Verification items for this drawing (mm, ordinates from the low corner). Round coordinates to 2 decimals unless told otherwise and drop trailing zeros. Loops run counter-clockwise (first coordinate to the right, second up) from the corner with the lowest first, then second, coordinate; pieces in that order, holes last. Notation, with made-up numbers: (13, -10) -> (42, -10) arc R23 ccw to (42, 2) -> close; hole circle Ø10 at (-32.5, 30.25). An arc over 180 degrees is marked (long way). Use a Markdown table: item, result. Add a question column.
Q1. Sectioned sample at C-C, the plane y = 427. Enter the section's corners in (x, z).
Q2. Gauge pin test, flat ends, axial feed: P1, Ø10, axis at y = 351, z = 122.5, coming from the -X side; P2, Ø8, axis at x = 520, z = 6, coming from the -Y side; P3, Ø8, axis at y = 516.5, z = 6, coming from the -X side. Record the tip position at first contact, or that the pin passes through.
Q3. Material ranges on L1, parallel to Z at x = 297, y = 231; L2, parallel to X at y = 310, z = 293.5, recorded low to high.
Q4. Sectioned sample at B-B, the plane z = 326. Enter the section's corners in (x, y).
Q5. Sectioned sample at A-A, the plane x = 649. Enter the section's corners in (y, z), then the cut area to 3 significant figures.
Q6. Sectioned sample at D-D, the plane z = 272. Enter the section's corners in (x, y).
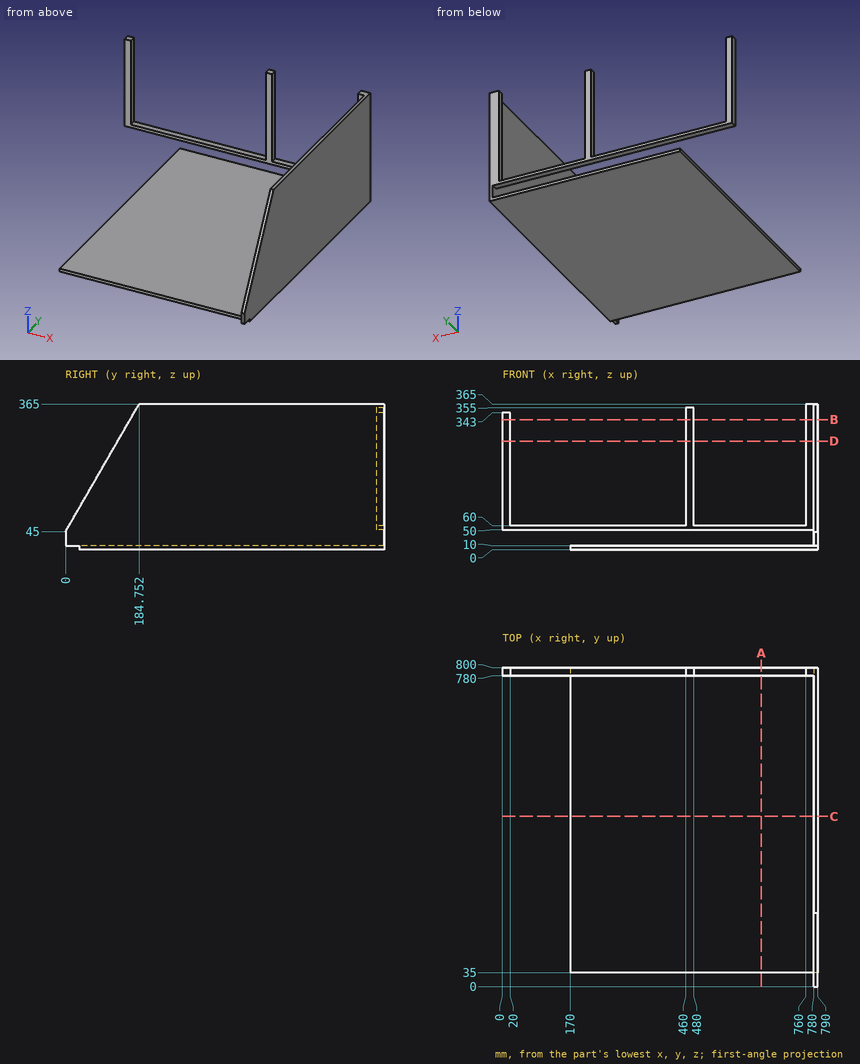
Values:
| question | item | result |
|---|---|---|
| 1 | outline | (170, 0) -> (790, 0) -> (790, 365) -> (780, 365) -> (780, 10) -> (170, 10) -> close |
| 2 | P1 | x = 780 |
| 2 | P2 | y = 35 |
| 2 | P3 | x = 170 |
| 3 | L1 | 0 to 10 |
| 3 | L2 | 780 to 790 |
| 4 | outline | (0, 780) -> (20, 780) -> (20, 800) -> (0, 800) -> close; (460, 780) -> (480, 780) -> (480, 800) -> (460, 800) -> close; (760, 780) -> (780, 780) -> (780, 162.24) -> (790, 162.24) -> (790, 800) -> (760, 800) -> close |
| 5 | outline | (35, 0) -> (800, 0) -> (800, 10) -> (35, 10) -> close; (780, 50) -> (800, 50) -> (800, 60) -> (780, 60) -> close |
| 5 | area | 7,850 mm^2 |
| 6 | outline | (0, 780) -> (20, 780) -> (20, 800) -> (0, 800) -> close; (460, 780) -> (480, 780) -> (480, 800) -> (460, 800) -> close; (760, 780) -> (780, 780) -> (780, 131.06) -> (790, 131.06) -> (790, 800) -> (760, 800) -> close |
